Check sheet for the modelled part. Datum: model origin and axes. Units: mm. A direction names the side the tool comes from. Give positions to 0.01 mm unless a question says otherwise; leave off trailing zeros. Order: outer loops, then holes, each group sorted by start corner. A loop starts at its lowest first (then second) coordinate and runs counter-clockwise, first axis right, second up.
from build123d import *

# Parameters (mm, degrees)
F0_R     = 40
F0_R_2   = 2.5
F1_DEPTH = 2.5


with BuildPart() as f1:
    # F0 (on Front) → F1 (new body, symmetric)
    with BuildSketch(Plane.XZ):
        Circle(F0_R)
        with BuildLine():
            Line((-5.59017, -5), (-5, -5))
            Line((-5, -5), (-5, -5.59017))
            Line((-5, -5.59017), (-5, -30.594117))
            ThreePointArc((-5, -30.594117), (-21.92031, -21.92031), (-30.594117, -5))
            Line((-30.594117, -5), (-5.59017, -5))
        make_face(mode=Mode.SUBTRACT)
        with BuildLine():
            Line((5, -30.594117), (5, -5.59017))
            Line((5, -5.59017), (5, -5))
            Line((5, -5), (5.59017, -5))
            Line((5.59017, -5), (30.594117, -5))
            ThreePointArc((30.594117, -5), (21.92031, -21.92031), (5, -30.594117))
        make_face(mode=Mode.SUBTRACT)
        with BuildLine():
            ThreePointArc((-30.594117, 5), (-21.92031, 21.92031), (-5, 30.594117))
            Line((-5, 30.594117), (-5, 5.59017))
            Line((-5, 5.59017), (-5, 5))
            Line((-5, 5), (-5.59017, 5))
            Line((-5.59017, 5), (-30.594117, 5))
        make_face(mode=Mode.SUBTRACT)
        Circle(F0_R_2, mode=Mode.SUBTRACT)
        with BuildLine():
            Line((5.59017, 5), (5, 5))
            Line((5, 5), (5, 5.59017))
            Line((5, 5.59017), (5, 30.594117))
            ThreePointArc((5, 30.594117), (21.92031, 21.92031), (30.594117, 5))
            Line((30.594117, 5), (5.59017, 5))
        make_face(mode=Mode.SUBTRACT)
    extrude(amount=F1_DEPTH, both=True)


solid = f1.part
1) Section check C-C, the plane z = 0. Record the cut outline in (x, y), then the cut area to 3 significant figures.
Recorded:
outline: (-40, -2.5) - (-2.5, -2.5) - (-2.5, 2.5) - (-40, 2.5) - close; (2.5, -2.5) - (40, -2.5) - (40, 2.5) - (2.5, 2.5) - close
area: 375 mm2
2) Section check B-B, the plane y = -0.8. Record the cut outline in (x, z).
Recorded:
outline: circle Ø80 at (0, 0); hole (-30.59, -5) arc R31 ccw to (-5, -30.59) - (-5, -5) - close; hole (-30.59, 5) - (-5, 5) - (-5, 30.59) arc R31 ccw to start; hole circle Ø5 at (0, 0); hole (5, -30.59) arc R31 ccw to (30.59, -5) - (5, -5) - close; hole (5, 5) - (30.59, 5) arc R31 ccw to (5, 30.59) - close
3) Draft check along Z on faces 3 (the face through (21.73, -0.04, 22.11)), 4 (the face through (-8.67, -0.04, -39.05)), 5 (the face through (-1, -2.5, -8)). Enter one of: +Z half, -Z half, draft (parallel to the pull), parting line (faces both ways), or undercut.
Recorded:
face 3: undercut
face 4: parting line
face 5: draft
4) Depth check by flat-ended pin: pin 1 Ø3 at (x, z) = (0, 0) entering from -Y; pin 2 Ø1.5 at (x, y) = (27, 1.5) entering from +Z; pin 3 Ø2.5 at (x, y) = (15.5, -0.5) entering from -Z; pin 4 Ø1 at (x, y) = (-18.5, -1.5) entering from +Z. Enter the tip coordinate at first touch or a pass-through.
Recorded:
pin 1: passes through
pin 2: stops at z = 30.18
pin 3: stops at z = -37.38
pin 4: stops at z = 35.72
5) Set-up check for faces 1 (the face through (22.11, -0.04, -21.73)), 2 (the face through (-1, 2.5, -8)): record each of +Z, -Z, +X, -X, +Y, -Y from which the full face is reachable in a straight line by a thin tool's end or side.
Recorded:
face 1: +Y, -Y
face 2: +Z, -Z, +X, -X, +Y
6) Material ranges on L1, parallel to Z at x = 0, y = 1.05; L2, parallel to X at y = -1.7, z = 17; L3, parallel to X at y = -1, z = 15, recorded low to high.
Recorded:
L1: z = -40 to -2.5, 2.5 to 40
L2: x = -36.21 to -25.92, -5 to 5, 25.92 to 36.21
L3: x = -37.08 to -27.13, -5 to 5, 27.13 to 37.08
7) Section check D-D, the plane x = 20.5. Record the cut outline in (y, z), then the cut area to 3 significant figures.
Recorded:
outline: (-2.5, -34.35) - (2.5, -34.35) - (2.5, -23.25) - (-2.5, -23.25) - close; (-2.5, -5) - (2.5, -5) - (2.5, 5) - (-2.5, 5) - close; (-2.5, 23.25) - (2.5, 23.25) - (2.5, 34.35) - (-2.5, 34.35) - close
area: 161 mm2
8) Section check A-A, the plane x = 0. Record the cut outline in (y, z), then the cut area to 3 significant figures.
Recorded:
outline: (-2.5, -40) - (2.5, -40) - (2.5, -2.5) - (-2.5, -2.5) - close; (-2.5, 2.5) - (2.5, 2.5) - (2.5, 40) - (-2.5, 40) - close
area: 375 mm2
